Check sheet for the modelled part. Datum: model origin and axes. Units: mm. Give positions to 0.01 mm unless a question says otherwise; leave off trailing zeros. Write each loop counter-clockwise with the first axis right and the second up, starting at its lowest first coordinate (ties: lowest second). Pieces come first, ordered by that corner, then holes. Notation, with made-up numbers: (-27, -4.5) -> (-22, -4.5) arc R24 cw to (-22, 33.5) -> close; hole circle Ø8 at (43.5, 70.5). An arc over 180 degrees is marked (long way). Use a Markdown table: item, result. Add a question column.
1. Scan lines: probe 1 along Y at (x, z) = (6, -57.5); probe 2 along Z at (x, y) = (10, 1849); probe 3 along Z at (x, y) = (0, 2256.5). Record each from-to range of solid material in increasing order. Write a range as [from, to].
2. Gauge pin test, flat ends, axial feed: P1, Ø22.5, axis at x = 1.5, y = 172, coming from the +Z side; P2, Ø4, axis at x = -14, y = 1783.5, coming from the +Z side. Record the tip position at first contact, or that the pin passes through.
3. Cross-section at B-B (y = 2132). Enter the section's corners in (x, z), then the cut area to 3 significant figures.
4. Cross-section at A-A (x = -0.5). Enter the section's corners in (y, z), then the cut area to 3 significant figures.
Solid Edge part; units mm, degrees
sketch "Sketch1" plane through (0, 0, 0) normal (0, -1, 0) x (1, 0, 0)
  line L0 (-22.5, -72.5) -> (22.5, -72.5)
  line L1 (22.5, -72.5) -> (22.5, 72.5)
  line L2 (22.5, 72.5) -> (-22.5, 72.5)
  line L3 (-22.5, 72.5) -> (-22.5, -72.5)
extrude "Protrusion1" add sketch "Sketch1" against normal blind 2370
sketch "Sketch2" plane through (22.5, 1185, 0) normal (1, 0, 0) x (0, 1, 0)
  line L0 (1035, 72.5) -> (1035, 36.25)
  line L1 (1035, 36.25) -> (990, 36.25)
  line L2 (990, 36.25) -> (990, 72.5)
  line L3 (990, 72.5) -> (1035, 72.5)
  line L4 (-1035, 72.5) -> (-1035, 36.25)
  line L5 (-1035, 36.25) -> (-990, 36.25)
  line L6 (-990, 36.25) -> (-990, 72.5)
  line L7 (-990, 72.5) -> (-1035, 72.5)
extrude "ExtrudedCutout_1" cut sketch "Sketch2" against normal blind 89.2118
mirror "Mirror1" about plane through (0, 0, 0) normal (0, 0, -1) of "ExtrudedCutout_1"
sketch "Sketch3" plane through (-22.5, 1185, 0) normal (-1, 0, 0) x (0, -1, 0)
  line L0 (-1185, -21.4815) -> (-508.4584, 75.4061)
  line L1 (-508.4584, 75.4061) -> (-1185, 75.4061)
  line L2 (-1185, 75.4061) -> (-1185, -21.4815)
extrude "ExtrudedCutout_3" cut sketch "Sketch3" against normal blind 291.9601
properties material "Wood, Pine"
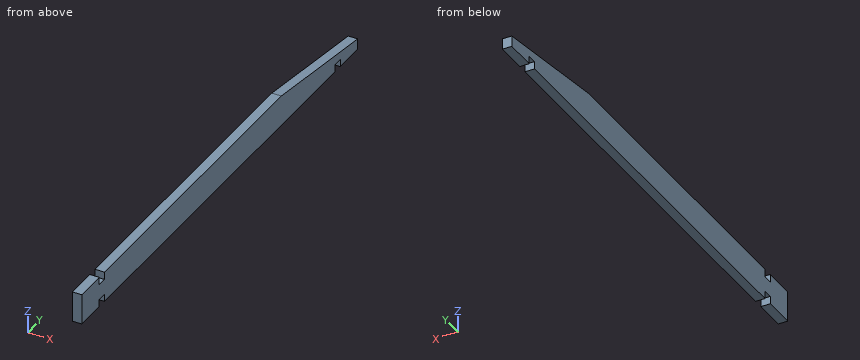
Worked answers:
| question | item | result |
|---|---|---|
| 1 | probe 1 | y = [0, 150], [195, 2175], [2220, 2370] |
| 1 | probe 2 | z = [-72.5, 53.13] |
| 1 | probe 3 | z = [-72.5, -5.23] |
| 2 | P1 | stops at z = 36.25 |
| 2 | P2 | stops at z = 62.8 |
| 3 | outline | (-22.5, -72.5) -> (22.5, -72.5) -> (22.5, 12.6) -> (-22.5, 12.6) -> close |
| 3 | area | 3,830 mm² |
| 4 | outline | (0, -72.5) -> (150, -72.5) -> (150, -36.25) -> (195, -36.25) -> (195, -72.5) -> (2175, -72.5) -> (2175, -36.25) -> (2220, -36.25) -> (2220, -72.5) -> (2370, -72.5) -> (2370, -21.48) -> (1713.75, 72.5) -> (195, 72.5) -> (195, 36.25) -> (150, 36.25) -> (150, 72.5) -> (0, 72.5) -> close |
| 4 | area | 308,000 mm² |
